Can you work these out from the model? Positions are in its coordinate system, mm. Face numbers are marked on the shaded views. A direction names the side the tool comes from. Give positions to 0.01 mm unless a question says otherwise; leave off trailing zeros. Loops run counter-clockwise (first coordinate to the right, second up) from the corner with the lowest first, then second, coordinate; pieces in that order, holes last. Notation, with made-up numbers: (15.25, 30.25) -> (48.25, 30.25) arc R14 cw to (48.25, 55.25) -> close; hole circle Ø10 at (44.25, 8). An arc over 180 degrees is marked (long way). One line per question, with ' | ' between items.
from build123d import *

# Parameters (mm, degrees)
SKETCH1_W           = 56
SKETCH1_H           = 56
SKETCH1_R           = 1.55
SKETCH1_W_2         = 30
SKETCH1_H_2         = 30
BOSS_EXTRUDE1_DEPTH = 5
SKETCH2_R           = 3.55
CUT_EXTRUDE1_DEPTH  = 3
FILLET1_R           = 5
SKETCH3_W           = 56
SKETCH3_H           = 56
SKETCH3_W_2         = 50
SKETCH3_H_2         = 50
BOSS_EXTRUDE2_DEPTH = 20
FILLET2_R           = 5


with BuildPart() as part:
    # Sketch1 → Boss-Extrude1 (new body)
    with BuildSketch(Plane(origin=(0, 0, 0), x_dir=(1, 0, 0), z_dir=(0, 1, 0))):
        Rectangle(SKETCH1_W, SKETCH1_H)
        with Locations((-20, 20)):
            Circle(SKETCH1_R, mode=Mode.SUBTRACT)
        with Locations((20, 20)):
            Circle(SKETCH1_R, mode=Mode.SUBTRACT)
        with Locations((20, -20)):
            Circle(SKETCH1_R, mode=Mode.SUBTRACT)
        with Locations((-20, -20)):
            Circle(SKETCH1_R, mode=Mode.SUBTRACT)
        Rectangle(SKETCH1_W_2, SKETCH1_H_2, mode=Mode.SUBTRACT)
    extrude(amount=BOSS_EXTRUDE1_DEPTH)

    # Sketch2 → Cut-Extrude1 (cut)
    with BuildSketch(Plane.XZ):
        with Locations((-20, 20)):
            Circle(SKETCH2_R)
        with Locations((20, 20)):
            Circle(SKETCH2_R)
        with Locations((-20, -20)):
            Circle(SKETCH2_R)
        with Locations((20, -20)):
            Circle(SKETCH2_R)
    extrude(amount=-CUT_EXTRUDE1_DEPTH, mode=Mode.SUBTRACT)

    # Fillet1
    fillet1_edges = [part.edges().sort_by_distance(p)[0] for p in [
        (15, 2.5, 15),
        (15, 2.5, -15),
        (-15, 2.5, -15),
        (-15, 2.5, 15),
    ]]
    fillet(fillet1_edges, radius=FILLET1_R)

    # Sketch3 → Boss-Extrude2 (add)
    with BuildSketch(Plane.XZ):
        Rectangle(SKETCH3_W, SKETCH3_H)
        Rectangle(SKETCH3_W_2, SKETCH3_H_2, mode=Mode.SUBTRACT)
    extrude(amount=BOSS_EXTRUDE2_DEPTH)

    # Fillet2
    fillet2_edges = [part.edges().sort_by_distance(p)[0] for p in [
        (-28, -7.5, -28),
        (28, -7.5, -28),
        (28, -7.5, 28),
        (-28, -7.5, 28),
    ]]
    fillet(fillet2_edges, radius=FILLET2_R)


solid = part.part
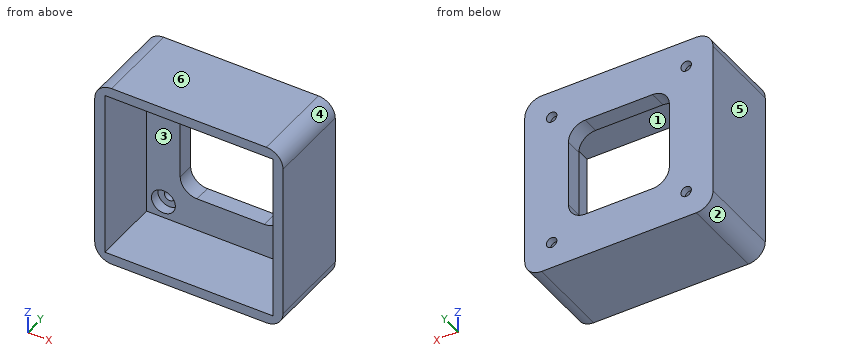
Q1. If we section it at B-B (y = 2): Write out the boundary of the cut face in (x, z), plus the area to 3 significant figures.
Entries:
outline: (-28, -23) arc R5 ccw to (-23, -28) -> (23, -28) arc R5 ccw to (28, -23) -> (28, 23) arc R5 ccw to (23, 28) -> (-23, 28) arc R5 ccw to (-28, 23) -> close; hole circle Ø7.1 at (-20, -20); hole circle Ø7.1 at (-20, 20); hole (-15, -10) arc R5 ccw to (-10, -15) -> (10, -15) arc R5 ccw to (15, -10) -> (15, 10) arc R5 ccw to (10, 15) -> (-10, 15) arc R5 ccw to (-15, 10) -> close; hole circle Ø7.1 at (20, -20); hole circle Ø7.1 at (20, 20) | area: 2,080 mm²
Q2. On a 3-axis mill with a long thin cutter (end or side, diameter ignored), from which of +Z, -Z, +X, -X, +Y, -Y can I reach the whole of each face in a straight line? I mean the marked faces 1 and 2. Say none if no direction works.
Entries:
face 1: -Y | face 2: -Z, -X, +Y, -Y
Q3. For pin 1 Ø3.5 at (x, z) = (-20.5, 19) entering from -Y; pin 2 Ø15 at (x, z) = (6, 0) entering from -Y; pin 3 Ø5 at (x, z) = (-1.5, -16) entering from -Y, each with a flat end and sliding along its axis, tell me the tip position at first contact or that it passes through.
Entries:
pin 1: y = 3 | pin 2: through | pin 3: y = 0
Q4. If we mould it in two halves opening along X, with no side actions, what happens to the marked faces 3, 4, 5 and 6? For each: pulls with the +X half, pulls with the -X half, needs draft (parallel to the pull), parting line crosses it, or undercut.
Entries:
face 3: undercut | face 4: pulls with the +X half | face 5: pulls with the -X half | face 6: needs draft
Q5. If we section it at D-D (z = 8): Write out the boundary of the cut face in (x, y), plus the area to 3 significant figures.
Entries:
outline: (-28, -20) -> (-25, -20) -> (-25, 0) -> (-15, 0) -> (-15, 5) -> (-28, 5) -> close; (15, 0) -> (25, 0) -> (25, -20) -> (28, -20) -> (28, 5) -> (15, 5) -> close | area: 250 mm²
Q6. If we section it at A-A (z = 20): Write out the boundary of the cut face in (x, y), plus the area to 3 significant figures.
Entries:
outline: (-28, -20) -> (-25, -20) -> (-25, 0) -> (-23.55, 0) -> (-23.55, 3) -> (-21.55, 3) -> (-21.55, 5) -> (-28, 5) -> close; (-18.45, 3) -> (-16.45, 3) -> (-16.45, 0) -> (16.45, 0) -> (16.45, 3) -> (18.45, 3) -> (18.45, 5) -> (-18.45, 5) -> close; (21.55, 3) -> (23.55, 3) -> (23.55, 0) -> (25, 0) -> (25, -20) -> (28, -20) -> (28, 5) -> (21.55, 5) -> close | area: 345 mm²
Q7. If we section it at C-C (x = -1): Write out the boundary of the cut face in (y, z), plus the area to 3 significant figures.
Entries:
outline: (-20, -28) -> (5, -28) -> (5, -15) -> (0, -15) -> (0, -25) -> (-20, -25) -> close; (-20, 25) -> (0, 25) -> (0, 15) -> (5, 15) -> (5, 28) -> (-20, 28) -> close | area: 250 mm²
Q8. If I drill on probe 1 along X at (y, z) = (4.25, 20); probe 2 along Z at (x, y) = (20, 1.7); probe 3 along Z at (x, y) = (-14, -17), over which ranges is the centre line in solid material (lowest first)? Write a range as from..to.
Entries:
probe 1: -28..-21.55, -18.45..18.45, 21.55..28 | probe 2: -28..-23.55, -16.45..16.45, 23.55..28 | probe 3: -28..-25, 25..28
